Could you check a few things on this model? Use its own coordinates, in mm. Face numbers are marked on the shaded views. A direction names the side the tool comes from. Coordinates: 2 decimals unless noted, no trailing zeros. Write each loop counter-clockwise with the first axis right and the second up, starting at its lowest first coordinate (ties: lowest second). Pieces come first, ordered by that corner, then holes. Notation, with made-up numbers: M 46,44 L 81,44 A32 ccw 81,80 Z; hole C 45,18.25 d7. An arc over 180 degrees is marked long. Answer as CSV lines item,"result". Start each with the question number.
Item 1: We'd pull the mould along Y, two halves only. Please class the marked faces 1, 2 and 3: +Y half, -Y half, draft (parallel to the pull), parting line (faces both ways), or undercut.
Item 2: Suppose I cut it at A-A, the plane z = 92.5. Write out the boundary of the cut face in (x, y).
Item 3: I'm going to push flat-ended pins straight in: P1, Ø13.5, axis at x = -55, z = 92.5, coming from the +Y side; P2, Ø10, axis at y = 25.5, z = -32, coming from the -X side; P3, Ø6.5, axis at y = 16, z = 70, coming from the -X side; P4, Ø4, axis at x = 22, y = -37.5, coming from the +Z side. Where does each tip first touch, or does it pass through?
Item 4: If I drill on line 1 along X through (y, z) = (14.5, -28.5); line 2 along Y through (x, z) = (-64.2, 92.5), over which ranges is the centre line in solid material (lowest first)? Write a range as [from, to].
Item 5: Suppose I cut it at B-B, the plane y = 24. Write out the boundary of the cut face in (x, z).
Item 6: Suppose I cut it at C-C, the plane x = 1. Write out the boundary of the cut face in (y, z).
Item 7: On a 3-axis mill with a long thin cutter (end or side, diameter ignored), from which of +Z, -Z, +X, -X, +Y, -Y can I reach the whole of each face in a straight line? I mean the marked faces 4, 5, 6 and 7. Say none if no direction works.
Item 8: Suppose I cut it at D-D, the plane z = 42. Write out the boundary of the cut face in (x, y), and give its area (3 significant figures).
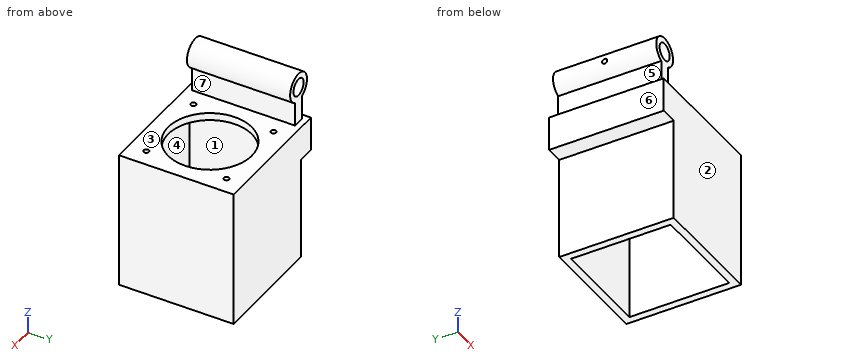
```python
from build123d import *

# Parameters (mm, degrees)
SKETCH1_W                           = 100
SKETCH1_H                           = 100
BOSS_EXTRUDE1_DEPTH                 = 60
SKETCH2_W                           = 87
SKETCH2_H                           = 87
CUT_EXTRUDE1_DEPTH                  = 113.5
SKETCH4_R                           = 36.55
CUT_EXTRUDE2_DEPTH                  = 6.5
F_4_6_4_6_DIAMETER_HOLE1_D          = 4.6
CIRPATTERN1_COUNT                   = 4
SKETCH13_W                          = 30
SKETCH13_H                          = 100
BOSS_EXTRUDE6_DEPTH                 = 15
BOSS_EXTRUDE7_DEPTH                 = 45
BOSS_EXTRUDE7_DEPTH_BACK            = 45
SKETCH15_R                          = 12.5
BOSS_EXTRUDE8_REACH                 = 148.48
BOSS_EXTRUDE8_END_RADIUS            = 12.5
SKETCH14_W                          = 10
SKETCH14_H                          = 90
SKETCH16_R                          = 7.5
CUT_EXTRUDE4_DEPTH                  = 90
CUT_EXTRUDE5_REACH                  = 165.554
CUT_EXTRUDE5_END_RADIUS             = 12.5
SKETCH17_R                          = 2.25
CUT_EXTRUDE5_DIRECTION_2_REACH      = 165.554
CUT_EXTRUDE5_DIRECTION_2_END_RADIUS = 7.5


with BuildPart() as part:
    # Sketch1 → Boss-Extrude1 (new, symmetric)
    with BuildSketch(Plane.XY):
        Rectangle(SKETCH1_W, SKETCH1_H)
    extrude(amount=BOSS_EXTRUDE1_DEPTH, both=True)

    # Sketch2 → Cut-Extrude1 (cut)
    with BuildSketch(Plane(origin=(0, 0, -60), x_dir=(-1, 0, 0), z_dir=(0, 0, -1))):
        Rectangle(SKETCH2_W, SKETCH2_H)
    extrude(amount=-CUT_EXTRUDE1_DEPTH, mode=Mode.SUBTRACT)

    # Sketch4 → Cut-Extrude2 (cut)
    with BuildSketch(Plane.XY.offset(60)):
        Circle(SKETCH4_R)
    extrude(amount=-CUT_EXTRUDE2_DEPTH, mode=Mode.SUBTRACT)

    # Ø4.6 (4.6) Diameter Hole1 (through all)
    with Locations(Plane.XY.offset(60)):
        with Locations((-35, 35)):
            f_4_6_4_6_diameter_hole1 = Hole(F_4_6_4_6_DIAMETER_HOLE1_D / 2)

    # CirPattern1: Ø4.6 (4.6) Diameter Hole1 ×4 about axis
    cirpattern1_axis = Axis((0, 0, 0), (0, 0, 1))
    for i in range(1, CIRPATTERN1_COUNT):
        add(f_4_6_4_6_diameter_hole1.rotate(cirpattern1_axis, i * 360 / CIRPATTERN1_COUNT), mode=Mode.SUBTRACT)

    # Sketch13 → Boss-Extrude6 (add)
    with BuildSketch(Plane.ZY.offset(50)):
        with Locations((45, 0)):
            Rectangle(SKETCH13_W, SKETCH13_H)
    extrude(amount=BOSS_EXTRUDE6_DEPTH)



with BuildPart() as body_2:
    # Sketch15 → Boss-Extrude7 (new, two sides: drawn at the far end of the back side and taken through both)
    with BuildSketch(Plane(origin=(0, 0, 0), x_dir=(1, 0, 0), z_dir=(0, 1, 0)).offset(-BOSS_EXTRUDE7_DEPTH_BACK)):
        with Locations(Location((-55, -92.5, 0), (0, 0, 270))):
            Circle(SKETCH15_R)
    extrude(amount=BOSS_EXTRUDE7_DEPTH + BOSS_EXTRUDE7_DEPTH_BACK)


with BuildPart() as part_1:
    add(part.part)

    add(body_2.part)  # Boss-Extrude8 merges body 2
    # Boss-Extrude8: up to this cylinder (the profile starts outside it)
    boss_extrude8_end = Plane(origin=(-55, 0, 92.5), z_dir=(0, -1, 0)) * Cylinder(BOSS_EXTRUDE8_END_RADIUS, 322.96, mode=Mode.PRIVATE)
    # Sketch14 → Boss-Extrude8 (add, up to the surface)
    with BuildSketch(Plane.XY.offset(60), mode=Mode.PRIVATE) as boss_extrude8_sk1:
        with Locations((-55, 0)):
            Rectangle(SKETCH14_W, SKETCH14_H)
    boss_extrude8_tool1 = extrude(boss_extrude8_sk1.sketch, amount=BOSS_EXTRUDE8_REACH, mode=Mode.PRIVATE) - boss_extrude8_end
    add(boss_extrude8_tool1.solids().sort_by_distance((-55, 0, 60))[0])

    # Sketch16 → Cut-Extrude4 (cut)
    with BuildSketch(Plane(origin=(0, 45, 0), x_dir=(1, 0, 0), z_dir=(0, 1, 0))):
        with Locations(Location((-55, -92.5, 0), (0, 0, 270))):
            Circle(SKETCH16_R)
    extrude(amount=-CUT_EXTRUDE4_DEPTH, mode=Mode.SUBTRACT)

    # Cut-Extrude5: up to this cylinder (the profile starts inside it)
    cut_extrude5_end = Plane(origin=(-55, 0, 92.5), z_dir=(0, -1, 0)) * Cylinder(CUT_EXTRUDE5_END_RADIUS, 357.108, mode=Mode.PRIVATE)
    # Sketch17 → Cut-Extrude5 (cut, up to the surface)
    with BuildSketch(Plane(origin=(-65, 0, 0), x_dir=(0, 0, -1), z_dir=(1, 0, 0)), mode=Mode.PRIVATE) as cut_extrude5_sk1:
        with Locations((-92.5, 0)):
            Circle(SKETCH17_R)
    cut_extrude5_tool1 = extrude(cut_extrude5_sk1.sketch, amount=-CUT_EXTRUDE5_REACH, mode=Mode.PRIVATE) & cut_extrude5_end
    add(cut_extrude5_tool1.solids().sort_by_distance((-65, 0, 92.5))[0], mode=Mode.SUBTRACT)

    # Cut-Extrude5 direction 2: up to this cylinder (the profile starts outside it)
    cut_extrude5_direction_2_end = Plane(origin=(-55, 0, 92.5), z_dir=(0, 1, 0)) * Cylinder(CUT_EXTRUDE5_DIRECTION_2_END_RADIUS, 347.108, mode=Mode.PRIVATE)
    # Sketch17 → Cut-Extrude5 direction 2 (cut, up to the surface)
    with BuildSketch(Plane(origin=(-65, 0, 0), x_dir=(0, 0, -1), z_dir=(1, 0, 0)), mode=Mode.PRIVATE) as cut_extrude5_direction_2_sk1:
        with Locations((-92.5, 0)):
            Circle(SKETCH17_R)
    cut_extrude5_direction_2_tool1 = extrude(cut_extrude5_direction_2_sk1.sketch, amount=CUT_EXTRUDE5_DIRECTION_2_REACH, mode=Mode.PRIVATE) - cut_extrude5_direction_2_end
    add(cut_extrude5_direction_2_tool1.solids().sort_by_distance((-65, 0, 92.5))[0], mode=Mode.SUBTRACT)


solid = part_1.part
```
Ans:
1,face 1,"undercut"
1,face 2,"-Y half"
1,face 3,"draft"
2,outline,"M -67.5,-45 L -62.5,-45 L -62.5,-2.25 L -67.5,-2.25 Z; M -67.5,2.25 L -62.5,2.25 L -62.5,45 L -67.5,45 Z; M -47.5,-45 L -42.5,-45 L -42.5,45 L -47.5,45 Z"
3,P1,"passes through"
3,P2,"stops at x = -50"
3,P3,"stops at x = -60"
3,P4,"stops at z = 60"
4,line 1,"x = [-50, -43.5], [43.5, 50]"
4,line 2,"y = [-45, -2.25], [2.25, 45]"
5,outline,"M -65,30 L -50,30 L -50,-60 L -43.5,-60 L -43.5,53.5 L -27.57,53.5 L -27.57,60 L -50,60 L -50,81.04 A12.5 ccw long -60,81.04 L -60,60 L -65,60 Z; M 27.57,53.5 L 43.5,53.5 L 43.5,-60 L 50,-60 L 50,60 L 27.57,60 Z; hole C -55,92.5 d15"
6,outline,"M -50,-60 L -43.5,-60 L -43.5,53.5 L -36.54,53.5 L -36.54,60 L -50,60 Z; M 36.54,53.5 L 43.5,53.5 L 43.5,-60 L 50,-60 L 50,60 L 36.54,60 Z"
7,face 4,"-Z"
7,face 5,"-X, +Y, -Y"
7,face 6,"-Z, -X, +Y, -Y"
7,face 7,"+X, +Y, -Y"
8,outline,"M -65,-50 L 50,-50 L 50,50 L -65,50 Z; hole M -43.5,-43.5 L 43.5,-43.5 L 43.5,43.5 L -43.5,43.5 Z"
8,area,"3,930 mm^2"
